from build123d import *

# Parameters (mm, degrees)
ESQUISSE1_W             = 80
ESQUISSE1_H             = 100
BOSS_EXTRU_1_DEPTH      = 20
ESQUISSE2_R             = 20
BOSS_EXTRU_2_DEPTH      = 30
ESQUISSE3_R             = 10
ENL_V_MAT_EXTRU_1_DEPTH = 82.240384046


with BuildPart() as part:
    # Esquisse1 → Boss.-Extru.1 (new body)
    with BuildSketch(Plane.XY):
        Rectangle(ESQUISSE1_W, ESQUISSE1_H)
    extrude(amount=BOSS_EXTRU_1_DEPTH)

    # Esquisse2 → Boss.-Extru.2 (add)
    with BuildSketch(Plane.XY.offset(20)):
        Circle(ESQUISSE2_R)
    extrude(amount=BOSS_EXTRU_2_DEPTH)

    # Esquisse3 → Enlèv. mat.-Extru.1 (cut, through all)
    with BuildSketch(Plane.XY.offset(50)):
        Circle(ESQUISSE3_R)
    extrude(amount=-ENL_V_MAT_EXTRU_1_DEPTH, mode=Mode.SUBTRACT)


solid = part.part
Geometry: final body of the model. Coordinates: model frame, mm. Coordinates: 2 decimals unless noted, no trailing zeros. Order: outer loops, then holes, each group sorted by start corner. A loop starts at its lowest first (then second) coordinate and runs counter-clockwise, first axis right, second up. Notation, with made-up numbers: M -24.5,53 L 34.5,53 A37 cw 34.5,91 Z; hole C 68,17 d3. An arc over 180 degrees is marked long. One line per question, with ' | ' between items. Start each with the question number.
Item 1: Ray query, probe 1 along Y at (x, z) = (0, 25); probe 2 along Z at (x, y) = (24, -44); probe 3 along X at (y, z) = (1, 47.5). Return the intervals inside material, ascending. Write a range as [from, to].
Item 2: Pin query (flat end, axial travel): pin 1 Ø1 at (y, z) = (-4.5, 28) entering from +X; pin 2 Ø2 at (y, z) = (-5, 38) entering from -X; pin 3 Ø1 at (x, z) = (-15, 42.5) entering from +Y (3 decimals). Return the tip coordinate at first contact, or that it passes through.
Item 3: Cut plane A-A, the plane y = 0. Return the cut outline in (x, z).
Item 4: Cut plane D-D, the plane y = 34. Return the cut outline in (x, z).
Item 5: Draft query along X for faces 1 (the cylindrical face through (-4.336, -19.524, 34.79)), 2 (the cylindrical face through (-2.17, -9.76, 25.35)), 3 (the flat face through (-1, 12, 0)). Return one class per face: released by +X, released by -X, zero draft, split by the parting line, or undercut.
Item 6: Cut plane C-C, the plane z = 34. Return the cut outline in (x, y), then the cut area to 3 significant figures.
Item 7: Cut plane B-B, the plane x = 0. Return the cut outline in (y, z).
A:
1) probe 1: y = [-20, -10], [10, 20] | probe 2: z = [0, 20] | probe 3: x = [-19.97, -9.95], [9.95, 19.97]
2) pin 1: stops at x = 19.6 | pin 2: stops at x = -19.6 | pin 3: stops at y = 13.775
3) outline: M -40,0 L -10,0 L -10,50 L -20,50 L -20,20 L -40,20 Z; M 10,0 L 40,0 L 40,20 L 20,20 L 20,50 L 10,50 Z
4) outline: M -40,0 L 40,0 L 40,20 L -40,20 Z
5) face 1: split by the parting line | face 2: undercut | face 3: zero draft
6) outline: C 0,0 d40; hole C 0,0 d20 | area: 942 mm2
7) outline: M -50,0 L -10,0 L -10,50 L -20,50 L -20,20 L -50,20 Z; M 10,0 L 50,0 L 50,20 L 20,20 L 20,50 L 10,50 Z
